from build123d import *

# Parameters (mm, degrees)
F0_W     = 152.4
F0_H     = 76.2
F1_DEPTH = 25.4
F2_W     = 76.2
F2_H     = 50.8
F3_DEPTH = 76.2


with BuildPart() as f1:
    # F0 (on Top) → F1 (new body)
    with BuildSketch(Plane.XY):
        with Locations((-76.2, 38.1)):
            Rectangle(F0_W, F0_H)
    extrude(amount=F1_DEPTH)

    # F2 (on Right) → F3 (join)
    with BuildSketch(Plane.YZ):
        with Locations((38.1, -25.4)):
            Rectangle(F2_W, F2_H)
    extrude(amount=-F3_DEPTH)


solid = f1.part
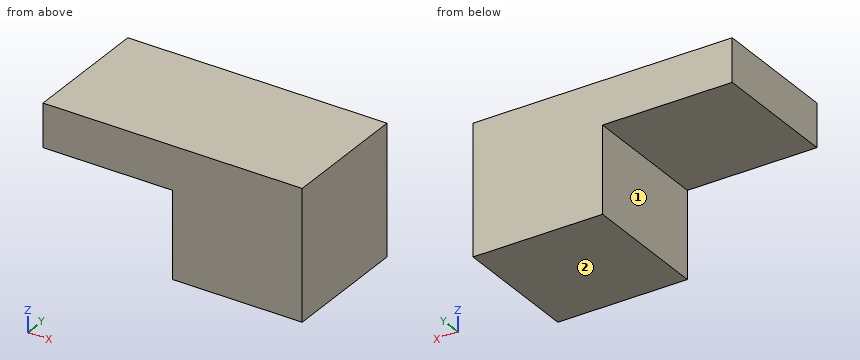
For this review, take the finished solid that the model builds, in its own axes (mm). Face numbers are marked on the shaded views. A direction names the side the tool comes from. Round coordinates to 2 decimals unless told otherwise and drop trailing zeros. Order: outer loops, then holes, each group sorted by start corner. A loop starts at its lowest first (then second) coordinate and runs counter-clockwise, first axis right, second up. Notation, with made-up numbers: M 56,3.25 L 109,3.25 A25 cw 109,35.25 Z; hole C 78,82 d10. An arc over 180 degrees is marked long. Use a Markdown table: item, result. Add a question column.
Item 1: Tool access review of the marked faces 1 and 2: name each direction out of +Z, -Z, +X, -X, +Y, -Y from which nothing blocks a thin tool from reaching the whole face with its end or side.
Item 2: Add section B-B, the plane z = -12. Give the boundary of the cut face in (x, y), then the cut area to 3 significant figures.
Item 3: To check wall thickness, follow line 1 along X through (y, z) = (54, -4); line 2 along Z through (x, y) = (-83, 64). State the ranges of each line that lie inside material, in increasing order.
Item 4: Add section C-C, the plane x = -111. Give the boundary of the cut face in (y, z).
Item 5: Add section A-A, the plane y = 51.5. Give the boundary of the cut face in (x, z).
Item 6: Insertion check: pin 1 (4 mm diameter, centred on y = 30, z = -7.5, fed in from -X); pin 2 (4 mm diameter, centred on x = -115, y = 13, fed in from -Z); pin 3 (12 mm diameter, centred on y = 46.5, z = -33, fed in from +X). Each pin has a flat end and moves straight along its axis. Give the tip position at first contact, or say it passes through.
Geometry results:
| question | item | result |
|---|---|---|
| 1 | face 1 | -Z, -X, +Y, -Y |
| 1 | face 2 | -Z, +X, -X, +Y, -Y |
| 2 | outline | M -76.2,0 L 0,0 L 0,76.2 L -76.2,76.2 Z |
| 2 | area | 5,810 mm² |
| 3 | line 1 | x = -76.2 to 0 |
| 3 | line 2 | z = 0 to 25.4 |
| 4 | outline | M 0,0 L 76.2,0 L 76.2,25.4 L 0,25.4 Z |
| 5 | outline | M -152.4,0 L -76.2,0 L -76.2,-50.8 L 0,-50.8 L 0,25.4 L -152.4,25.4 Z |
| 6 | pin 1 | stops at x = -76.2 |
| 6 | pin 2 | stops at z = 0 |
| 6 | pin 3 | stops at x = 0 |
